from build123d import *

# Parameters (mm, degrees)
SKETCH1_R           = 1.5
BOSS_EXTRUDE1_DEPTH = 3
BOSS_EXTRUDE2_START = 3
SKETCH1_4_R         = 1.5
SKETCH1_4_R_2       = 16
SKETCH1_4_R_3       = 13
BOSS_EXTRUDE2_DEPTH = 2
SKETCH1_5_R         = 6.1
CUT_EXTRUDE1_DEPTH  = 10


with BuildPart() as part:
    # Sketch1 → Boss-Extrude1 (new body)
    with BuildSketch(Plane(origin=(0, 0, 0), x_dir=(1, 0, 0), z_dir=(0, 1, 0))):
        with BuildLine():
            ThreePointArc((19.8125, 2.732186624), (14.142135624, 14.142135624), (2.732186624, 19.8125))
            ThreePointArc((2.732186624, 19.8125), (0, 25.5), (-2.732186624, 19.8125))
            ThreePointArc((-2.732186624, 19.8125), (-14.142135624, 14.142135624), (-19.8125, 2.732186624))
            ThreePointArc((-19.8125, 2.732186624), (-25.5, 0), (-19.8125, -2.732186624))
            ThreePointArc((-19.8125, -2.732186624), (-14.142135624, -14.142135624), (-2.732186624, -19.8125))
            ThreePointArc((-2.732186624, -19.8125), (0, -25.5), (2.732186624, -19.8125))
            ThreePointArc((2.732186624, -19.8125), (14.142135624, -14.142135624), (19.8125, -2.732186624))
            ThreePointArc((19.8125, -2.732186624), (25.5, 0), (19.8125, 2.732186624))
        make_face()
        with Locations((22, 0)):
            Circle(SKETCH1_R, mode=Mode.SUBTRACT)
        with Locations((0, 22)):
            Circle(SKETCH1_R, mode=Mode.SUBTRACT)
        with Locations((0, -22)):
            Circle(SKETCH1_R, mode=Mode.SUBTRACT)
        with Locations((-22, 0)):
            Circle(SKETCH1_R, mode=Mode.SUBTRACT)
    extrude(amount=BOSS_EXTRUDE1_DEPTH)

    # Sketch1_4 → Boss-Extrude2 (add)
    with BuildSketch(Plane(origin=(0, 0, 0), x_dir=(1, 0, 0), z_dir=(0, 1, 0)).offset(BOSS_EXTRUDE2_START)):
        with BuildLine():
            ThreePointArc((-2.732186624, -19.8125), (0, -25.5), (2.732186624, -19.8125))
            ThreePointArc((2.732186624, -19.8125), (0, -20), (-2.732186624, -19.8125))
        make_face()
        with Locations((0, -22)):
            Circle(SKETCH1_4_R, mode=Mode.SUBTRACT)
        with BuildLine():
            ThreePointArc((19.8125, 2.732186624), (19.953069939, 1.369306394), (20, 0))
            ThreePointArc((20, 0), (19.953069939, -1.369306394), (19.8125, -2.732186624))
            ThreePointArc((19.8125, -2.732186624), (25.5, 0), (19.8125, 2.732186624))
        make_face()
        with Locations((22, 0)):
            Circle(SKETCH1_4_R, mode=Mode.SUBTRACT)
        with BuildLine():
            ThreePointArc((-2.732186624, 19.8125), (0, 20), (2.732186624, 19.8125))
            ThreePointArc((2.732186624, 19.8125), (0, 25.5), (-2.732186624, 19.8125))
        make_face()
        with Locations((0, 22)):
            Circle(SKETCH1_4_R, mode=Mode.SUBTRACT)
        with BuildLine():
            ThreePointArc((-19.8125, -2.732186624), (-20, 0), (-19.8125, 2.732186624))
            ThreePointArc((-19.8125, 2.732186624), (-25.5, 0), (-19.8125, -2.732186624))
        make_face()
        with Locations((-22, 0)):
            Circle(SKETCH1_4_R, mode=Mode.SUBTRACT)
        Circle(SKETCH1_4_R_2)
        Circle(SKETCH1_4_R_3, mode=Mode.SUBTRACT)
    extrude(amount=BOSS_EXTRUDE2_DEPTH)

    # Sketch1_5 → Cut-Extrude1 (cut)
    with BuildSketch(Plane(origin=(0, 0, 0), x_dir=(1, 0, 0), z_dir=(0, 1, 0))):
        Circle(SKETCH1_5_R)
    extrude(amount=CUT_EXTRUDE1_DEPTH, mode=Mode.SUBTRACT)


solid = part.part
Build history of the part. All positions in model axes, mm. A direction names the side the tool comes from. Give positions to 0.01 mm unless a question says otherwise; leave off trailing zeros. Order: outer loops, then holes, each group sorted by start corner. A loop starts at its lowest first (then second) coordinate and runs counter-clockwise, first axis right, second up. Notation, with made-up numbers: M 38.25,-21 L 96.25,-21 A24 cw 96.25,-6 Z; hole C 21.5,-10 d6. An arc over 180 degrees is marked long. Put each result on its own line as item: value.
Item 1: Pull direction X, two halves, no side cores. Call faces 3 (the face through (-24, 5, 0)), 4 (the face through (-8.98, 3, -13.43)): +X half, -X half, draft (parallel to the pull), parting line (faces both ways), or undercut.
Results are:
face 3: draft
face 4: undercut
Item 2: Cut at C-C on z = -22. Write the cut outline in (x, y), then the cut area to 3 significant figures.
Results are:
outline: M -3.5,0 L -1.5,0 L -1.5,5 L -3.5,5 Z; M 1.5,0 L 3.5,0 L 3.5,5 L 1.5,5 Z
area: 20.0 mm2
Item 3: Drop flat-ended pins along their axis: pin 1 Ø1.8 at (x, z) = (-22, 0) entering from +Y; pin 2 Ø5 at (x, z) = (-16, 10) entering from +Y; pin 3 Ø1 at (y, z) = (1, -7.5) entering from +X (3 decimals); pin 4 Ø1.5 at (x, y) = (8, 1) entering from -Z. Give the stop position or say it passes through.
Results are:
pin 1: through
pin 2: y = 3
pin 3: x = 18.735
pin 4: z = -18.64
Item 4: Cut at D-D on x = -22. Write the cut outline in (y, z).
Results are:
outline: M 0,-3.5 L 5,-3.5 L 5,-1.5 L 0,-1.5 Z; M 0,1.5 L 5,1.5 L 5,3.5 L 0,3.5 Z
Item 5: Cut at B-B on y = 3.9. Count the separate pieces of the cut face and the enclosed holes in it, then the cut area to 3 significant figures.
Results are:
separate pieces: 5
enclosed holes: 5
area: 376 mm2
Item 6: Which spindle directions (+Z, -Z, +X, -X, +Y, -Y) get a long thin tool onto all of the face, cutting with end or side? Do faces 1 (the face through (0, 4, 20)), 2 (the face through (20.5, 2.46, -0.07)). Say none if no direction does.
Results are:
face 1: +Y
face 2: +Y, -Y
Item 7: Cut at A-A on x = 0. Write the cut outline in (y, z), then the cut area to 3 significant figures.
Results are:
outline: M 0,-25.5 L 5,-25.5 L 5,-23.5 L 0,-23.5 Z; M 0,-20.5 L 5,-20.5 L 5,-20 L 3,-20 L 3,-16 L 5,-16 L 5,-13 L 3,-13 L 3,-6.1 L 0,-6.1 Z; M 0,6.1 L 3,6.1 L 3,13 L 5,13 L 5,16 L 3,16 L 3,20 L 5,20 L 5,20.5 L 0,20.5 Z; M 0,23.5 L 5,23.5 L 5,25.5 L 0,25.5 Z
area: 120 mm2
Item 8: Wall check: probe 1 along Z at (x, y) = (22, 1.4); probe 2 along X at (y, z) = (0.6, 4); probe 3 along X at (y, z) = (3.8, 3). Give the ranges that are in metal, low to high.
Results are:
probe 1: -3.5 to -1.5, 1.5 to 3.5
probe 2: -19.6 to -4.61, 4.61 to 19.6
probe 3: -23.8 to -20.2, -15.72 to -12.65, 12.65 to 15.72, 20.2 to 23.8
